Build history of the part. All positions in model axes, mm. Face numbers are marked on the shaded views. A direction names the side the tool comes from. Coordinates: 2 decimals unless noted, no trailing zeros. Order: outer loops, then holes, each group sorted by start corner. A loop starts at its lowest first (then second) coordinate and runs counter-clockwise, first axis right, second up. Notation, with made-up numbers: (-35.5, 19) -> (1.5, 19) arc R10 ccw to (1.5, 34) -> close; hole circle Ø7 at (-8.5, 36). An arc over 180 degrees is marked (long way). Write each question's results on one line, items separated by ' | '.
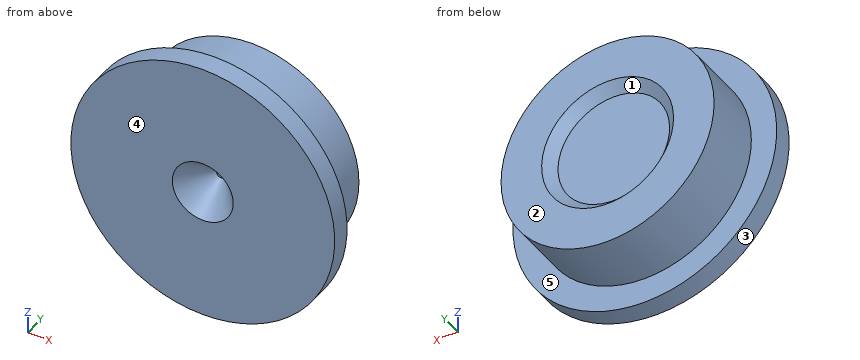
from build123d import *

# Parameters (mm, degrees)
BASES_R             = 6.5
BASE_DEPTH          = 1
O_RINGCAPTURES_R    = 5.25
O_RINGCAPTURE_DEPTH = 3
TOPBORES_R          = 3.25
TOPBORE_DEPTH       = 0.5
CHAMFER1_SIZE       = 0.5
CYLINDERBORES_R     = 1.5
CUT_EXTRUDE1_DEPTH  = 1.5
CUT_EXTRUDE1_DRAFT  = -40


with BuildPart() as part:
    # BaseS → Base (new body)
    with BuildSketch(Plane(origin=(0, 0, 0), x_dir=(1, 0, 0), z_dir=(0, 1, 0))):
        with Locations(Location((0, 0, 0), (0, 0, 270))):
            Circle(BASES_R)
    extrude(amount=-BASE_DEPTH)

    # O-RingCaptureS → O-RingCapture (add)
    with BuildSketch(Plane(origin=(0, 0, 0), x_dir=(1, 0, 0), z_dir=(0, 1, 0))):
        with Locations(Location((0, 0, 0), (0, 0, 270))):
            Circle(O_RINGCAPTURES_R)
    extrude(amount=O_RINGCAPTURE_DEPTH)

    # TopBoreS → TopBore (cut)
    with BuildSketch(Plane(origin=(0, 3, 0), x_dir=(1, 0, 0), z_dir=(0, 1, 0))):
        with Locations(Location((0, 0, 0), (0, 0, 270))):
            Circle(TOPBORES_R)
    extrude(amount=-TOPBORE_DEPTH, mode=Mode.SUBTRACT)

    # Chamfer1
    chamfer1_edges = [part.edges().sort_by_distance(p)[0] for p in [
        (0, 2.5, -3.25),
    ]]
    chamfer(chamfer1_edges, length=CHAMFER1_SIZE - 0.0001)  # a hair under: the kernel refuses the full size


with BuildPart() as cut_extrude1_tool:
    # CylinderBoreS → Cut-Extrude1 (with draft: the straight prism first)
    with BuildSketch(Plane(origin=(0, -1, 0), x_dir=(-1, 0, 0), z_dir=(0, -1, 0))):
        Circle(CYLINDERBORES_R)
    extrude(amount=-CUT_EXTRUDE1_DEPTH)
    # Cut-Extrude1: the draft: its side faces are tilted about the plane it starts from
    cut_extrude1_sides = [cut_extrude1_tool.faces().sort_by_distance(p)[0] for p in [
        (1.5, -0.25, 0),
    ]]
    draft(cut_extrude1_sides, Plane(origin=(0, -1, 0), x_dir=(-1, 0, 0), z_dir=(0, -1, 0)), CUT_EXTRUDE1_DRAFT)


with BuildPart() as part_1:
    add(part.part)

    # Cut-Extrude1: cut by cut_extrude1_tool
    add(cut_extrude1_tool.part, mode=Mode.SUBTRACT)


solid = part_1.part
Item 1: Slice it at C-C, the plane y = 1.95. List the corners of the cut face in (x, z).
Answer:
outline: circle Ø10.5 at (0, 0)
Item 2: Pull direction Z, two halves, no side cores. Call the marked faces 1, 2 and 3: released by +Z, released by -Z, zero draft, split by the parting line, or undercut.
Answer:
face 1: undercut | face 2: zero draft | face 3: split by the parting line
Item 3: Drill centre lines: line 1 (Y direction, x = 1.5, z = -1); line 2 (Z direction, x = -0.5, y = 0.1); line 3 (Z direction, x = -2, y = 2.05). Where is each one in solid material? Low to high. Write a range as from..to.
Answer:
line 1: y = -1..2.5 | line 2: z = -5.23..-0.29, 0.29..5.23 | line 3: z = -4.85..4.85
Item 4: Pin check, flat tip, straight feed: pin 1 (2 mm diameter, centred on y = 0.5, z = -4, fed in from -X). Stop position of the tip, or through.
Answer:
pin 1: stops at x = -5.69
Item 5: Slice it at D-D, the plane y = 2.7. List the corners of the cut face in (x, z), and give its area (3 significant figures).
Answer:
outline: circle Ø10.5 at (0, 0); hole circle Ø5.9 at (0, 0) | area: 59.2 mm^2
Item 6: Tool access for the marked faces 4 and 5: list every direction of +Z, -Z, +X, -X, +Y, -Y with a clear straight run to the whole face (end or side of a thin tool).
Answer:
face 4: +Z, -Z, +X, -X, -Y | face 5: +Y
